Build history of the part. All positions in model axes, mm. A direction names the side the tool comes from. Give positions to 0.01 mm unless a question says otherwise; leave off trailing zeros. Order: outer loops, then holes, each group sorted by start corner. A loop starts at its lowest first (then second) coordinate and runs counter-clockwise, first axis right, second up. Notation, with made-up numbers: (33.25, 82.5) - (39.25, 82.5) arc R18 cw to (39.25, 97.5) - close; hole circle Ø2 at (4.25, 68.5). An arc over 180 degrees is marked (long way). Use a Markdown table: item, result. Add a question column.
(1) Wall check: line 1 (Y direction, x = 0, z = 12.5) (3 decimals); line 2 (Y direction, x = -2.5, z = 4.25); line 3 (X direction, y = -22, z = 13). Give the ranges that are in metal, low to high.
(2) Which spindle directions (+Z, -Z, +X, -X, +Y, -Y) get a long thin tool onto all of the face, cutting with end or side? Do faces 4 (the face through (10.683, -21.819, 16.064)), 5 (the face through (-0.41, -22.25, 12.86)). Say none if no direction does.
(3) Slice it at A-A (x = 0). Write the cut outline in (y, z) (3 decimals).
(4) Slice it at D-D (x = -8.5). Write the cut outline in (y, z), then the cut area to 3 significant figures.
(5) Slice it at C-C (z = 12.7). Write the cut outline in (x, y) (3 decimals).
(6) Mould opens along Y. For faces 1 (the face through (3, -3, 25.4)), 2 (the face through (0, -38.1, 13)), 3 (the face through (-0.69, -3.1, 12.52)) say: +Y half, -Y half, draft (parallel to the pull), parting line (faces both ways), or undercut.
(7) Slice it at B-B (y = 0). Write the cut outline in (x, z) (3 decimals).
(8) Flat gauge pins, fed straight in: pin 1 (5.5 mm diameter, centred on x = 0, y = 0, fed in from -Z); pin 2 (3 mm diameter, centred on y = -31, z = 17.5, fed in from -X); pin 3 (6 mm diameter, centred on x = 9.5, z = 17.5, fed in from +Y); pin 4 (2 mm diameter, centred on y = -4, z = 16.5, fed in from +X). Where does each tip first touch, or does it go through?
from build123d import *

# Parameters (mm, degrees)
F0_R          = 12.7
F1_DEPTH      = 25.4
F2_R          = 11.2
F3_DEPTH      = 38.1
F4_R          = 3.175
F5_DEPTH      = 25.4
F5_DEPTH_BACK = 25.4
F7_R          = 3.175
F8_DEPTH      = 12.7


with BuildPart() as f1:
    # F0 (on Top) → F1 (new body)
    with BuildSketch(Plane.XY):
        Circle(F0_R)
    extrude(amount=F1_DEPTH)

    # F2 (on Front) → F3 (join)
    with BuildSketch(Plane.XZ):
        with Locations((0, 12.7)):
            Circle(F2_R)
    extrude(amount=F3_DEPTH)

    # F4 (on Top) → F5 (cut, two sides)
    with BuildSketch(Plane.XY) as f5_sk:
        Circle(F4_R)
    extrude(amount=-F5_DEPTH, mode=Mode.SUBTRACT)
    extrude(f5_sk.sketch, amount=F5_DEPTH_BACK, mode=Mode.SUBTRACT)

    # F7 (on offset) → F8 (cut, symmetric)
    with BuildSketch(Plane.XY.offset(12.7)):
        with Locations((0, -25.4)):
            Circle(F7_R)
    extrude(amount=F8_DEPTH, both=True, mode=Mode.SUBTRACT)


solid = f1.part
Solution:
| question | item | result |
|---|---|---|
| 1 | line 1 | -38.1 to -28.575, -22.225 to -3.175, 3.175 to 12.7 |
| 1 | line 2 | -38.1 to -27.36, -23.44 to -1.96, 1.96 to 12.45 |
| 1 | line 3 | -11.2 to 11.2 |
| 2 | face 4 | -Y |
| 2 | face 5 | +Z, -Z |
| 3 | outline | (-38.1, 1.5) - (-28.575, 1.5) - (-28.575, 23.9) - (-38.1, 23.9) - close; (-22.225, 1.5) - (-12.7, 1.5) - (-12.7, 0) - (-3.175, 0) - (-3.175, 25.4) - (-12.7, 25.4) - (-12.7, 23.9) - (-22.225, 23.9) - close; (3.175, 0) - (12.7, 0) - (12.7, 25.4) - (3.175, 25.4) - close |
| 4 | outline | (-38.1, 5.41) - (-9.44, 5.41) - (-9.44, 0) - (9.44, 0) - (9.44, 25.4) - (-9.44, 25.4) - (-9.44, 19.99) - (-38.1, 19.99) - close |
| 4 | area | 897 mm2 |
| 5 | outline | (-11.2, -38.1) - (11.2, -38.1) - (11.2, -5.987) arc R12.7 ccw (long way) to (-11.2, -5.987) - close; hole circle Ø6.35 at (0, -25.4); hole circle Ø6.35 at (0, 0) |
| 6 | face 1 | draft |
| 6 | face 2 | -Y half |
| 6 | face 3 | undercut |
| 7 | outline | (-12.7, 0) - (-3.175, 0) - (-3.175, 25.4) - (-12.7, 25.4) - close; (3.175, 0) - (12.7, 0) - (12.7, 25.4) - (3.175, 25.4) - close |
| 8 | pin 1 | through |
| 8 | pin 2 | x = -10.7 |
| 8 | pin 3 | y = 10.91 |
| 8 | pin 4 | x = 12.34 |
